```python
from build123d import *

# Parameters (mm, degrees)
SKETCH1_R           = 8
BOSS_EXTRUDE1_DEPTH = 16
SKETCH2_R           = 5.6
CUT_EXTRUDE1_DEPTH  = 12
BOSS_EXTRUDE2_START = -6
BOSS_EXTRUDE2_DEPTH = 6


with BuildPart() as part:
    # Sketch1 → Boss-Extrude1 (new body)
    with BuildSketch(Plane(origin=(0, 0, 0), x_dir=(1, 0, 0), z_dir=(0, 1, 0))):
        with Locations(Location((0, 0, 0), (0, 0, 270))):
            Circle(SKETCH1_R)
    extrude(amount=BOSS_EXTRUDE1_DEPTH)

    # Sketch2 → Cut-Extrude1 (cut)
    with BuildSketch(Plane.XZ):
        with Locations(Location((0, 0, 0), (0, 0, 270))):
            Circle(SKETCH2_R)
    extrude(amount=-CUT_EXTRUDE1_DEPTH, mode=Mode.SUBTRACT)

    # Sketch4 → Boss-Extrude2 (add)
    with BuildSketch(Plane(origin=(0, 16, 0), x_dir=(1, 0, 0), z_dir=(0, 1, 0)).offset(BOSS_EXTRUDE2_START)):
        with BuildLine():
            Line((7.598545919, 10.426973043), (4.330349084, 7.158776209))
            ThreePointArc((4.330349084, 7.158776209), (4.05115191, 7.017889357), (3.742866535, 7.070427858))
            ThreePointArc((3.742866535, 7.070427858), (-5.656854249, -5.656854249), (7.070427858, 3.742866535))
            ThreePointArc((7.070427858, 3.742866535), (7.017889357, 4.05115191), (7.158776209, 4.330349084))
            Line((7.158776209, 4.330349084), (10.426973043, 7.598545919))
            Line((10.426973043, 7.598545919), (11.696836602, 6.32868236))
            Line((11.696836602, 6.32868236), (11.841186606, 11.841186606))
            Line((11.841186606, 11.841186606), (6.325753712, 11.699765249))
            Line((6.325753712, 11.699765249), (7.598545919, 10.426973043))
        make_face()
    extrude(amount=BOSS_EXTRUDE2_DEPTH)


solid = part.part
```
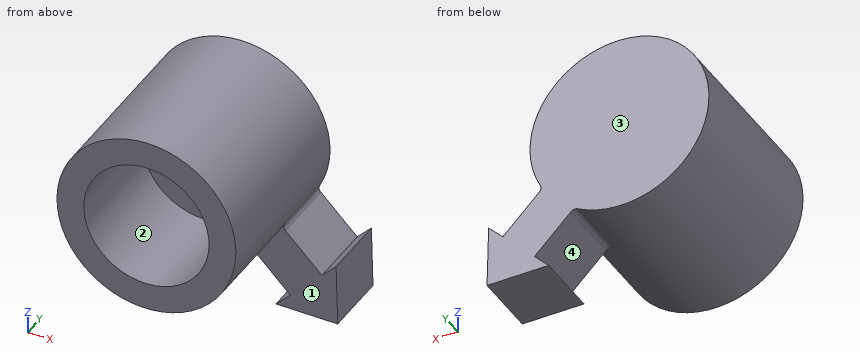
Model file for the job. Use its own axes, mm. Face numbers are marked on the shaded views. A direction names the side the tool comes from. Give positions to 0.01 mm unless a question says otherwise; leave off trailing zeros. Order: outer loops, then holes, each group sorted by start corner. A loop starts at its lowest first (then second) coordinate and runs counter-clockwise, first axis right, second up.
1) Saw through at D-D, the plane y = 11. Write the cut outline in (x, z), then the cut area to 3 significant figures.
2) 3-axis set-ups, long thin cutter, end or side, ignore diameter. For the marked faces 3 and 4: which of +Z, -Z, +X, -X, +Y, -Y reach the whole face in a straight line?
3) Mould opens along X. For the marked faces 1 and 2 say: +X half, -X half, draft (parallel to the pull), parting line (faces both ways), or undercut.
4) Saw through at B-B, the plane z = 0. Write the cut outline in (x, y), then the cut area to 3 significant figures.
5) Pin check, flat tips, straight feed: pin 1 (5 mm diameter, centred on x = 8, y = 9, fed in from +Z); pin 2 (5 mm diameter, centred on y = 13.5, z = -5.5, fed in from +X); pin 3 (1.5 mm diameter, centred on x = 4, z = -8, fed in from -Y); pin 4 (4 mm diameter, centred on x = 1, y = 2, fed in from -Z). Stop position of each tip, or through.
6) Wall check: probe 1 along X at (y, z) = (3.5, 0); probe 2 along Z at (x, y) = (-0.25, 3.5); probe 3 along Z at (x, y) = (-5, 5.5) (3 decimals). Give the ranges that are in metal, low to high.
7) Saw through at A-A, the plane x = 0. Write the cut outline in (y, z).
8) Saw through at C-C, the plane y = 8.5. Write the cut outline in (x, z), then the cut area to 3 significant figures.
Computed:
1. outline: (3.74, -7.07) arc R0.5 cw to (4.33, -7.16) - (7.6, -10.43) - (6.33, -11.7) - (11.84, -11.84) - (11.7, -6.33) - (10.43, -7.6) - (7.16, -4.33) arc R0.5 cw to (7.07, -3.74) arc R8 ccw (long way) to start
1. area: 236 mm2
2. face 3: +Z, -Z, +X, -X, +Y
2. face 4: +Y, -Y
3. face 1: draft
3. face 2: undercut
4. outline: (-8, 0) - (-5.6, 0) - (-5.6, 10) - (5.6, 10) - (5.6, 0) - (8, 0) - (8, 16) - (-8, 16) - close
4. area: 144 mm2
5. pin 1: stops at z = 5.81
5. pin 2: stops at x = 11.74
5. pin 3: passes through
5. pin 4: stops at z = -8
6. probe 1: x = -8 to -5.6, 5.6 to 8
6. probe 2: z = -8 to -5.59, 5.59 to 8
6. probe 3: z = -6.245 to -2.522, 2.522 to 6.245
7. outline: (0, -8) - (16, -8) - (16, 8) - (0, 8) - (0, 5.6) - (10, 5.6) - (10, -5.6) - (0, -5.6) - close
8. outline: circle Ø16 at (0, 0); hole circle Ø11.2 at (0, 0)
8. area: 103 mm2
